```python
from build123d import *

# Parameters (mm, degrees)
SKETCH_1_R                                = 3
EXTRUDE_1_DEPTH                           = 10.5
SKETCH_3_R                                = 1.5
EXTRUDE_2_DEPTH                           = 13
SKETCH_4_R                                = 3
EXTRUDE_3_DEPTH                           = 2
SKETCH_5_R                                = 1.5
EXTRUDE_4_DEPTH                           = 38.5
EXTRUDE_START                             = 29.5
SKETCH_7_R                                = 3
EXTRUDE_5_DEPTH                           = 2
EXTRUDE_START_2                           = 34
SKETCH_8_R                                = 3
EXTRUDE_6_DEPTH                           = 2
SKETCH_9_R                                = 3
EXTRUDE_7_DEPTH                           = 4
FILLET_1_R                                = 3
CUT_EXTRUDE_START                         = -8.5
CUT_EXTRUDE_1_DEPTH                       = 52.211239739
MIRROR_START                              = -8.5
MIRROR_2_AT_THE_SECOND_PLANE_COPY_1_DEPTH = 52.211239739


with BuildPart() as part:
    # 草图1 → 凸台-拉伸1 (new body)
    with BuildSketch(Plane.XY):
        with Locations(Location((0, 0, 0), (0, 0, 180))):
            Circle(SKETCH_1_R)
    extrude(amount=EXTRUDE_1_DEPTH)

    # 草图3 → 凸台-拉伸2 (add)
    with BuildSketch(Plane.XY):
        with Locations(Location((0, 0, 0), (0, 0, 180))):
            Circle(SKETCH_3_R)
    extrude(amount=EXTRUDE_2_DEPTH)

    # 草图4 → 凸台-拉伸3 (add)
    with BuildSketch(Plane.XY.offset(13)):
        with Locations(Location((0, 0, 0), (0, 0, 180))):
            Circle(SKETCH_4_R)
    extrude(amount=EXTRUDE_3_DEPTH)

    # 草图5 → 凸台-拉伸4 (add)
    with BuildSketch(Plane.XY):
        with Locations(Location((0, 0, 0), (0, 0, 180))):
            Circle(SKETCH_5_R)
    extrude(amount=EXTRUDE_4_DEPTH)

    # 草图7 → 凸台-拉伸5 (add)
    with BuildSketch(Plane.XY.offset(EXTRUDE_START)):
        with Locations(Location((0, 0, 0), (0, 0, 180))):
            Circle(SKETCH_7_R)
    extrude(amount=EXTRUDE_5_DEPTH)

    # 草图8 → 凸台-拉伸6 (add)
    with BuildSketch(Plane.XY.offset(EXTRUDE_START_2)):
        with Locations(Location((0, 0, 0), (0, 0, 180))):
            Circle(SKETCH_8_R)
    extrude(amount=EXTRUDE_6_DEPTH)

    # 草图9 → 凸台-拉伸7 (add)
    with BuildSketch(Plane.XY.offset(38.5)):
        with Locations(Location((0, 0, 0), (0, 0, 180))):
            Circle(SKETCH_9_R)
    extrude(amount=EXTRUDE_7_DEPTH)

    # 圆角1
    fillet_1_edges = [part.edges().sort_by_distance(p)[0] for p in [
        (3, 0, 42.5),
    ]]
    fillet(fillet_1_edges, radius=FILLET_1_R)

    # 草图10 → 切除-拉伸1 (cut)
    with BuildSketch(Plane(origin=(0, 0, 0), x_dir=(-1, 0, 0), z_dir=(0, 0, -1)).offset(CUT_EXTRUDE_START)):
        Polygon((-26.96639908, 1), (-2.828427125, 1), (-1, 1), (-1, 2.828427125), (-1, 26.96639908), (-35.136247307, 61.102646386), (-61.102646386, 35.136247307), align=None)
    cut_extrude_1 = extrude(amount=CUT_EXTRUDE_1_DEPTH, mode=Mode.SUBTRACT)

    # 镜向2: 切除-拉伸1 across plane
    add(cut_extrude_1.mirror(Plane.ZX), mode=Mode.SUBTRACT)

    # 镜向2 at the second plane: 切除-拉伸1 across plane
    add(cut_extrude_1.mirror(Plane(origin=(0, 0, 0), x_dir=(0, 0, 1), z_dir=(1, 0, 0))), mode=Mode.SUBTRACT)

    # 镜向2 at the second plane copy 1 sket → 镜向2 at the second plane copy 1 (cut)
    with BuildSketch(Plane(origin=(0, 0, 0), x_dir=(1, 0, 0), z_dir=(0, 0, -1)).offset(MIRROR_START)):
        Polygon((-26.96639908, 1), (-2.828427125, 1), (-1, 1), (-1, 2.828427125), (-1, 26.96639908), (-35.136247307, 61.102646386), (-61.102646386, 35.136247307), align=None)
    extrude(amount=MIRROR_2_AT_THE_SECOND_PLANE_COPY_1_DEPTH, mode=Mode.SUBTRACT)


solid = part.part
```
Input: part model. Units: mm. Frame: model coordinates. A direction names the side the tool comes from. Give positions to 0.01 mm unless a question says otherwise; leave off trailing zeros. Order: outer loops, then holes, each group sorted by start corner. A loop starts at its lowest first (then second) coordinate and runs counter-clockwise, first axis right, second up. Notation, with made-up numbers: (-0.5, -31) - (13.5, -31) arc R22 ccw to (13.5, 2) - close; hole circle Ø6 at (-16, -4.5). An arc over 180 degrees is marked (long way). Use a Markdown table: item, result.
(1) Line query: line 1 (Z direction, x = 2.2, y = -0.4); line 2 (Z direction, x = -1.05, y = -2.2); line 3 (X direction, y = 1.3, z = 7.5). Output: solid intervals per line, ascending. Write a range as from..to.
Computed values:
| item | result |
|---|---|
| line 1 | z = 0..10.5, 13..15, 29.5..31.5, 34..36, 38.5..41.5 |
| line 2 | z = 8.5..10.5, 13..15, 29.5..31.5, 34..36, 38.5..41.25 |
| line 3 | x = -1..1 |
(2) Access query for faces 1 (the flat face through (-1, -2, 4)), 2 (the flat face through (-1, 2, 4)), 3 (the flat face through (2, 1, 4)), 4 (the flat face through (-1.3, 1.3, 13)), 5 (the flat face through (1, -2, 4)). Directions: +Z, -Z, +X, -X, +Y, -Y. A direction counts if a zero-diameter tool reaches every point of the face in a straight line with its end or side. Return the directions, or none.
Computed values:
| item | result |
|---|---|
| face 1 | -Z, -X, -Y |
| face 2 | -Z, -X, +Y |
| face 3 | -Z, +X, +Y |
| face 4 | none |
| face 5 | -Z, +X, -Y |
(3) Section query A-A (y = -2.05). Output: boundary loops of the cut face in (x, z), then the cut area to 3 significant figures.
Computed values:
| item | result |
|---|---|
| outline | (-2.19, 8.5) - (-1, 8.5) - (-1, 0) - (1, 0) - (1, 8.5) - (2.19, 8.5) - (2.19, 10.5) - (-2.19, 10.5) - close; (-2.19, 13) - (2.19, 13) - (2.19, 15) - (-2.19, 15) - close; (-2.19, 29.5) - (2.19, 29.5) - (2.19, 31.5) - (-2.19, 31.5) - close; (-2.19, 34) - (2.19, 34) - (2.19, 36) - (-2.19, 36) - close; (-2.19, 38.5) - (2.19, 38.5) - (2.19, 39.5) arc R2.19 ccw to (-2.19, 39.5) - close |
| area | 64.0 mm2 |
(4) Section query D-D (z = 23.5). Output: boundary loops of the cut face in (x, y).
Computed values:
| item | result |
|---|---|
| outline | circle Ø3 at (0, 0) |
(5) Section query C-C (z = 7.5). Output: boundary loops of the cut face in (x, y), then the cut area to 3 significant figures.
Computed values:
| item | result |
|---|---|
| outline | (-2.83, -1) - (-1, -1) - (-1, -2.83) arc R3 ccw to (1, -2.83) - (1, -1) - (2.83, -1) arc R3 ccw to (2.83, 1) - (1, 1) - (1, 2.83) arc R3 ccw to (-1, 2.83) - (-1, 1) - (-2.83, 1) arc R3 ccw to start |
| area | 19.5 mm2 |
(6) Section query B-B (x = 2.3). Output: boundary loops of the cut face in (y, z).
Computed values:
| item | result |
|---|---|
| outline | (-1.93, 8.5) - (-1, 8.5) - (-1, 0) - (1, 0) - (1, 8.5) - (1.93, 8.5) - (1.93, 10.5) - (-1.93, 10.5) - close; (-1.93, 13) - (1.93, 13) - (1.93, 15) - (-1.93, 15) - close; (-1.93, 29.5) - (1.93, 29.5) - (1.93, 31.5) - (-1.93, 31.5) - close; (-1.93, 34) - (1.93, 34) - (1.93, 36) - (-1.93, 36) - close; (-1.93, 38.5) - (1.93, 38.5) - (1.93, 39.5) arc R1.93 ccw to (-1.93, 39.5) - close |
(7) Pin query (flat end, axial travel): pin 1 (1.5 mm diameter, centred on x = 2, z = 6, fed in from +Y); pin 2 (2 mm diameter, centred on y = 0, z = 21, fed in from +X); pin 3 (1 mm diameter, centred on y = 1.5, z = 19, fed in from -X). Return the tip coordinate at first contact, or that it passes through.
Computed values:
| item | result |
|---|---|
| pin 1 | stops at y = 1 |
| pin 2 | stops at x = 1.5 |
| pin 3 | stops at x = -1.12 |
(8) Draft query along Z for faces 6 (the flat face through (2, -2, 8.5)), 7 (the flat face through (2, -1, 4)), 8 (the cylindrical face through (-1.43, -0.45, 11.73)). Return one class per face: released by +Z, released by -Z, zero draft, split by the parting line, or undercut.
Computed values:
| item | result |
|---|---|
| face 6 | released by -Z |
| face 7 | zero draft |
| face 8 | undercut |
